Part model, mm, in its own coordinate system. Round coordinates to 2 decimals unless told otherwise and drop trailing zeros. Loops run counter-clockwise (first coordinate to the right, second up) from the corner with the lowest first, then second, coordinate; pieces in that order, holes last.
1) Band-saw the part on C-C, the plane z = 5.4. Write the cut outline in (x, y).
2) Mould opens along Y. For faces 1 (the flat face through (37, 6.042, 4)), 2 (the flat face through (70, -27, 4)), 3 (the cylindrical face through (14.253, -56.458, 4.479)) say: +Y half, -Y half, draft (parallel to the pull), parting line (faces both ways), or undercut.
3) Band-saw the part on A-A, the plane x = 39.5. Write the cut outline in (y, z).
4) Band-saw the part on D-D, the plane y = -15.5. Write the cut outline in (x, z), then the cut area to 3 significant figures.
5) Probe line 1 (X direction, y = 1, z = 5.6); line 2 (Y direction, x = 58.5, z = 4.85); line 3 (X direction, y = -7, z = 5.6). List the from-to ranges inside material, lowest first.
6) Band-saw the part on B-B, the plane y = -24. Write the cut outline in (x, z).
7) Drop flat-ended pins along their axis: P1, Ø2.5, axis at x = 14.45, y = -54.97, coming from the -Z side; P2, Ø10, axis at x = 37.5, y = -9.5, coming from the +Z side. Give the stop position or say it passes through.
Autodesk Inventor part; units mm, degrees
ref_plane "作業平面4" through (0, 0, 3) normal (0, 0, 1) x (1, 0, 0)
ref_plane "作業平面1" through (0, 0, 3) normal (0, 0, 1) x (1, 0, 0)
ref_plane "YZ Plane" through (0, 0, 0) normal (1, 0, 0) x (0, 1, 0)
sketch "ギア線図" plane through (0, 0, 0) normal (0, 0, 1) x (1, 0, 0)
  circle A0 centre (11.2246, -29.111) radius 11.1
  circle A1 centre (54.569, -27.2294) radius 20.05
  circle A2 centre (54.569, -27.2294) radius 4.55
  circle A3 centre (36.0807, -10.2532) radius 11.1
  circle A4 centre (39.569, -43.72) radius 2.05
  circle A5 centre (69.569, -43.72) radius 2.05
  circle A6 centre (72.4026, -13.8541) radius 2.05
  circle A7 centre (39.569, -43.72) radius 15
  circle A8 centre (69.569, -43.72) radius 15
  circle A9 centre (72.4026, -13.8541) radius 15
  circle A10 centre (54.569, -27.2294) radius 5.5 construction
  circle A11 centre (11.2246, -29.111) radius 13 construction
  circle A12 centre (54.569, -27.2294) radius 20.5 construction
  circle A13 centre (36.0807, -10.2532) radius 20.55
  circle A14 centre (36.0807, -10.2532) radius 21.5 construction
  circle A15 centre (36.0807, -10.2532) radius 13 construction
  circle A16 centre (39.569, -43.72) radius 2.5 construction
  circle A17 centre (69.569, -43.72) radius 2.5 construction
  circle A18 centre (72.4026, -13.8541) radius 2.5 construction
  circle A19 centre (11.2246, -29.111) radius 20.1
  circle A20 centre (11.2246, -29.111) radius 22 construction
  line L0 (39.569, -43.72) -> (69.569, -43.72)
  circle A21 centre (0, 0) radius 20.1
  circle A22 centre (0, 0) radius 22 construction
  circle A23 centre (39.569, -43.72) radius 9.5 construction
  circle A24 centre (69.569, -43.72) radius 9.5 construction
  circle A25 centre (72.4026, -13.8541) radius 9.5 construction
  line L1 (54.569, -27.2294) -> (39.569, -43.72)
  line L2 (39.569, -43.72) -> (33.651, -38.3369)
  circle A26 centre (33.651, -38.3369) radius 2.25
  point P0 (58.2233, -20.0465)
  point P1 (42.0436, -35)
  point P2 (21.5995, 15.2696)
  point P3 (38.2329, 5.9161)
  point P4 (24.1755, 8.4229)
  point P5 (21.6039, 15.1272)
  point P6 (23.3458, 16.3469)
  point P7 (23.3177, 16.3886)
  dimension "d7" = 22.2
  dimension "d8" = 40.1
  dimension "d9" = 9.1
  dimension "d11" = 22.2
  dimension "d12" = 4.1
  dimension "d13" = 4.1
  dimension "d14" = 4.1
  dimension "d15" = 30
  dimension "d16" = 30
  dimension "d17" = 30
  dimension "d18" = 11
  dimension "d21" = 26
  dimension "d29" = 41
  dimension "d39" = 22.2921
  dimension "d40" = 22.2921
  dimension "d41" = 22.2921
  dimension "d43" = 41.1
  dimension "d44" = 43
  dimension "d45" = 26
  dimension "d46" = 5
  dimension "d47" = 5
  dimension "d48" = 5
  dimension "d49" = 40.2
  dimension "d50" = 44
  dimension "d53" = 40.2
  dimension "d55" = 44
  dimension "d58" = 19
  dimension "d59" = 19
  dimension "d60" = 19
  dimension "d90" = 8
  dimension "d91" = 4.5
ref_plane "作業平面4" through (0, 0, 3) normal (0, 0, 1) x (1, 0, 0)
sketch "スケッチ5" plane through (0, 0, 3) normal (0, 0, 1) x (1, 0, 0)
  circle A0 centre (10.6068, -54.0855) radius 1.5
  circle A1 centre (23.1948, 12.8161) radius 1.5
  circle A2 centre (59.3303, 1.1874) radius 1.5
  circle A3 centre (54.3074, -26.8895) radius 5
  circle A4 centre (35.8191, -9.9133) radius 5
  point P0 (0, 0)
ref_plane "作業平面1" through (0, 0, 3) normal (0, 0, 1) x (1, 0, 0)
sketch "スケッチ6" plane through (0, 0, 3) normal (0, 0, 1) x (1, 0, 0)
  circle A0 centre (59.3303, 1.1874) radius 1.5
  line L0 (3.3835, -58.1874) -> (70, -58.1874)
  line L1 (70, -58.1874) -> (70, 6.042)
  line L2 (70, 6.042) -> (3.3835, 6.042)
  line L3 (3.3835, 6.042) -> (3.3835, -58.1874)
  circle A1 centre (11.2246, -29.111) radius 11.1
  circle A2 centre (36.0807, -10.2532) radius 11.1
  circle A3 centre (54.569, -27.2294) radius 4.55
  circle A4 centre (11.2246, -29.111) radius 6
  circle A5 centre (36.0807, -10.2532) radius 6
  circle A6 centre (54.569, -27.2294) radius 6
  circle A7 centre (14.4482, -54.9706) radius 1.5
  circle A8 centre (23.1948, 12.8161) radius 1.5
  circle A9 centre (59.3303, 1.1874) radius 1.5
  circle A10 centre (54.3074, -26.8895) radius 5
  circle A11 centre (35.8191, -9.9133) radius 5
  point P0 (0, 0)
  point P1 (0, 0)
  dimension "d85" = 12
  dimension "d86" = 12
  dimension "d87" = 12
extrude "押し出し3" add sketch "スケッチ6" along normal blind 3 contours L3 A1 L2 L1 L0 | L3 A1 | A2 picked at (3.9972, -29.111)
equation "\"d40\" = d39"
equation "\"d41\" = d40"
properties part number "アームフレーム改" material "アルミニウム 2014-T4"
Reported:
1. outline: (3.38, -58.19) - (70, -58.19) - (70, 6.04) - (3.38, 6.04) - close; hole circle Ø12 at (11.22, -29.11); hole circle Ø3 at (14.45, -54.97); hole circle Ø12 at (36.08, -10.25); hole circle Ø12 at (54.57, -27.23); hole circle Ø3 at (59.33, 1.19)
2. face 1: +Y half
2. face 2: draft
2. face 3: undercut
3. outline: (-58.19, 3) - (-15.18, 3) - (-15.18, 6) - (-58.19, 6) - close; (-5.32, 3) - (6.04, 3) - (6.04, 6) - (-5.32, 6) - close
4. outline: (3.38, 3) - (33.17, 3) - (33.17, 6) - (3.38, 6) - close; (38.99, 3) - (70, 3) - (70, 6) - (38.99, 6) - close
4. area: 182 mm2
5. line 1: x = 3.38 to 57.84, 60.82 to 70
5. line 2: y = -58.19 to -31.76, -22.7 to -0.06, 2.44 to 6.04
5. line 3: x = 3.38 to 31.04, 41.12 to 70
6. outline: (3.38, 3) - (8.08, 3) - (8.08, 6) - (3.38, 6) - close; (14.37, 3) - (49.51, 3) - (49.51, 6) - (14.37, 6) - close; (59.63, 3) - (70, 3) - (70, 6) - (59.63, 6) - close
7. P1: passes through
7. P2: stops at z = 6
